Here's how the part is built. I have some questions about the finished solid (model axes, mm). A direction names the side the tool comes from. Round coordinates to 2 decimals unless told otherwise and drop trailing zeros. Loops run counter-clockwise (first coordinate to the right, second up) from the corner with the lowest first, then second, coordinate; pieces in that order, holes last. Notation, with made-up numbers: M 38,20 L 91,20 A28 ccw 91,51 Z; hole C 42,-28 d9. An arc over 180 degrees is marked long. Use a Markdown table: item, result.
```python
from build123d import *

# Parameters (mm, degrees)
F0_W     = 101.6
F0_H     = 50.8
F1_DEPTH = 25.4
F2_R     = 11.6399110946
F3_DEPTH = 6.35


# Not quite as in the source:
# - a feature of the source that left no trace in its solid (it failed there, or was rolled back) is left out


with BuildPart() as f1:
    # F0 (on Front) → F1 (new body)
    with BuildSketch(Plane.XZ):
        with Locations((-1.7657391727, 1.1206692427)):
            Rectangle(F0_W, F0_H)
    extrude(amount=F1_DEPTH)

    # F2 (on face) → F3 (join)
    with BuildSketch(Plane.XZ.offset(25.4)):
        Circle(F2_R)
    extrude(amount=F3_DEPTH)


solid = f1.part
```
Q1. Imagine slicing it at D-D, the plane x = -20. Please give me the cut outline in (y, z), then the cut area to 3 significant figures.
Return value:
| item | result |
|---|---|
| outline | M -25.4,-24.28 L 0,-24.28 L 0,26.52 L -25.4,26.52 Z |
| area | 1,290 mm^2 |
Q2. For faces 1 (the flat face through (0, -31.75, 0)), 2 (the cylindrical face through (11.1, -28.5, 3.5)), which set-ups out of +Z, -Z, +X, -X, +Y, -Y let a thin tool reach every point of the face, with its end or its side?
Return value:
| item | result |
|---|---|
| face 1 | +Z, -Z, +X, -X, -Y |
| face 2 | -Y |
Q3. Imagine slicing it at A-A, the plane x = 0. Please give me the cut outline in (y, z).
Return value:
| item | result |
|---|---|
| outline | M -31.75,-11.64 L -25.4,-11.64 L -25.4,-24.28 L 0,-24.28 L 0,26.52 L -25.4,26.52 L -25.4,11.64 L -31.75,11.64 Z |
Q4. Will this pin go through, and if not, where does the flat tip stop? P1, Ø12, axis at x = 19.5, z = 10.5, coming from the -Y side.
Return value:
| item | result |
|---|---|
| P1 | stops at y = -25.4 |
Q5. Imagine slicing it at B-B, the plane z = 4. Please give me the cut outline in (x, y).
Return value:
| item | result |
|---|---|
| outline | M -52.57,-25.4 L -10.93,-25.4 L -10.93,-31.75 L 10.93,-31.75 L 10.93,-25.4 L 49.03,-25.4 L 49.03,0 L -52.57,0 Z |
Q6. Imagine slicing it at C-C, the plane y = -26.5. Please give me the cut outline in (x, z).
Return value:
| item | result |
|---|---|
| outline | C 0,0 d23.28 |
Q7. I need wall thicknesses on line 1 (Y direction, x = 29, z = 8); line 2 (Z direction, x = 6, y = -27); line 3 (Z direction, x = -10, y = -28.5). Which ranges of each line are inside material? Lowest first, please. Write a range as from..to.
Return value:
| item | result |
|---|---|
| line 1 | y = -25.4..0 |
| line 2 | z = -9.97..9.97 |
| line 3 | z = -5.96..5.96 |
